from build123d import *

# Parameters (mm, degrees)
SKETCH1_R             = 11.0998
BOSS_EXTRUDE1_DEPTH   = 3.175
F_8_CLEARANCE_HOLE2_D = 4.4958


with BuildPart() as part:
    # Sketch1 → Boss-Extrude1 (new body)
    with BuildSketch(Plane.XY):
        with BuildLine():
            Line((-188.264639147, 81.011774484), (56.809800323, 298.704514086))
            ThreePointArc((56.809800323, 298.704514086), (76.096805757, 305.388436009), (94.461024604, 296.476710194))
            Line((94.461024604, 296.476710194), (260.194034881, 109.897568099))
            ThreePointArc((260.194034881, 109.897568099), (271.059668812, 38.975929697), (210.82, 0))
            Line((210.82, 0), (-157.48, 0))
            ThreePointArc((-157.48, 0), (-200.811863601, 29.88880366), (-188.264639147, 81.011774484))
        make_face()
        with Locations((-157.48, 46.355)):
            Circle(SKETCH1_R, mode=Mode.SUBTRACT)
        with Locations((74.521510517, 278.765)):
            Circle(SKETCH1_R, mode=Mode.SUBTRACT)
        with Locations((210.82, 66.04)):
            Circle(SKETCH1_R, mode=Mode.SUBTRACT)
    extrude(amount=BOSS_EXTRUDE1_DEPTH)

    # #8 Clearance Hole2 (through all)
    with Locations(Plane.XY.offset(3.175)):
        with Locations((17.768914495, 247.038768822), (36.758927911, 263.907064244), (110.26846103, 259.557542359), (127.136756453, 240.567528943), (208.528289616, 148.938453927), (225.396585039, 129.948440511), (270.394698688, 62.514995218), (253.027203769, 23.832796231), (172.72, 12.7), (147.32, 12.7), (-93.98, 12.7), (-119.38, 12.7), (-194.875991874, 32.144446994), (-151.345471312, 96.81921091), (-132.355457896, 113.687506333), (-68.58, 149.225), (-68.58, 92.075), (121.92, 92.075), (121.92, 149.225), (71.12, 200.025), (26.67, 120.65), (0.55626, 75.2475), (56.43626, 75.2475), (56.43626, 17.4625), (0.55626, 17.4625)):
            Hole(F_8_CLEARANCE_HOLE2_D / 2)


solid = part.part
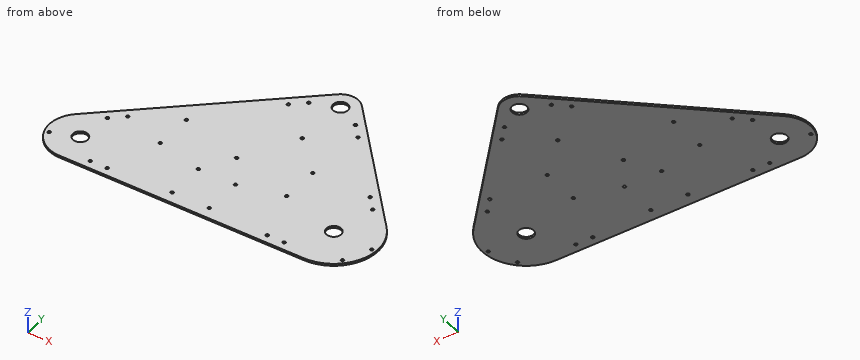
Here's how the part is built. I have some questions about the finished solid (model axes, mm). Give positions to 0.01 mm unless a question says otherwise; leave off trailing zeros. Order: outer loops, then holes, each group sorted by start corner. A loop starts at its lowest first (then second) coordinate and runs counter-clockwise, first axis right, second up. Notation, with made-up numbers: (59.5, -2.75) -> (73.5, -2.75) arc R22 cw to (73.5, 24.25) -> close; hole circle Ø3 at (73.25, 51). An arc over 180 degrees is marked (long way). One line per item, written item: value. Start each with the question number.
1. I need wall thicknesses on probe 1 along Y at (x, z) = (121.92, 1.2); probe 2 along X at (y, z) = (149.5, 0.5); probe 3 along X at (y, z) = (64, 3.05). Which ranges of each line are inside material? Lowest first, please. Write a range as from..to.
2. Imagine slicing it at A-A, the plane z = 0.65. Count the separate pieces of the cut face and the enclosed holes in it, plus the area to 3 significant figures.
3. Imagine slicing it at B-B, the plane y = 186. List the corners of the cut face in (x, z) for me (3 decimals), plus the area to 3 significant figures.
4. Imagine slicing it at C-C, the plane y = 232.5. List the corners of the cut face in (x, z) for me (3 decimals), plus the area to 3 significant figures.
5. Will these pins go through, and if not, where does the flat tip stop? pin 1 Ø20 at (x, y) = (-157.48, 46.355) entering from +Z; pin 2 Ø1.5 at (y, z) = (104, 2) entering from -X.
Values follow:
1. probe 1: y = 0..89.83, 94.32..146.98, 151.47..265.56
1. probe 2: x = -111.16..-70.81, -66.35..119.69, 124.15..206.35, 210.7..225.02
1. probe 3: x = -200.35..199.91, 221.73..268.71, 272.08..276.83
2. separate pieces: 1
2. enclosed holes: 28
2. area: 91,400 mm2
3. outline: (-70.071, 0) -> (192.594, 0) -> (192.594, 3.175) -> (-70.071, 3.175) -> close
3. area: 834 mm2
4. outline: (-17.722, 0) -> (151.29, 0) -> (151.29, 3.175) -> (-17.722, 3.175) -> close
4. area: 537 mm2
5. pin 1: passes through
5. pin 2: stops at x = -163.23
